The listing builds one solid part. Answer for the finished solid, in the listing's coordinates (mm). Face numbers are marked on the shaded views. A direction names the side the tool comes from. Coordinates: 2 decimals unless noted, no trailing zeros. Loops run counter-clockwise (first coordinate to the right, second up) from the corner with the lowest first, then second, coordinate; pieces in that order, holes last. Notation, with made-up numbers: M -31.5,-22 L -22.5,-22 A34 cw -22.5,12 Z; hole C -34,-24 d1. An arc over 180 degrees is marked long. Answer as a JSON object with one key per item and string values. Group by question number.
1. Determine the mould class of the marked faces 3, 4 and 5 for opening direction Y: released by +Y, released by -Y, zero draft, split by the parting line, or undercut.
2. For the marked faces 1 and 2, determine the directions among +Z, -Z, +X, -X, +Y, -Y from which every point of the face is accessible in a straight line to the end or side of a thin tool.
3. A cutting plane is placed at A-A on z = 10. Give the vertices of the cut face in (x, y), and give its area (4 significant figures).
4. A cutting plane is placed at C-C on y = 10. Give the vertices of the cut face in (x, z), and give its area (3 significant figures).
5. Straight lines are drawn through the part: L1, parallel to X at y = 6, z = 3.75; L2, parallel to Y at x = 67.5, z = 9.5; L3, parallel to Z at x = 10, y = 3.5. For each, find the intervals that lie inside material, in ascending order.
6. A cutting plane is placed at B-B on x = 45. Give the vertices of the cut face in (y, z), and give its area (3 significant figures).
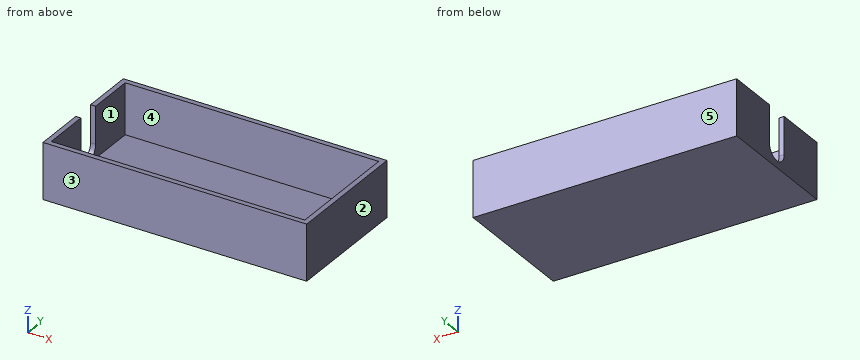
from build123d import *

# Parameters (mm, degrees)
ESQUISSE1_W             = 75
ESQUISSE1_H             = 35
BOSS_EXTRU_1_DEPTH      = 15
COQUE1_T                = 1.5
ENL_V_MAT_EXTRU_1_DEPTH = 15


with BuildPart() as part:
    # Esquisse1 → Boss.-Extru.1 (new body)
    with BuildSketch(Plane.XY):
        with Locations((37.5, 17.5)):
            Rectangle(ESQUISSE1_W, ESQUISSE1_H)
    extrude(amount=BOSS_EXTRU_1_DEPTH)

    # Coque1
    coque1_openings = [part.faces().sort_by_distance(p)[0] for p in [
        (37.5, 17.5, 15),
    ]]
    offset(amount=COQUE1_T, openings=coque1_openings, kind=Kind.INTERSECTION)

    # Esquisse2 → Enlèv. mat.-Extru.1 (cut)
    with BuildSketch(Plane.ZY.offset(1.5)):
        with BuildLine():
            Line((4, 21), (15.502923277, 21))
            ThreePointArc((15.502923277, 21), (19.002923277, 17.5), (15.502923277, 14))
            Line((15.502923277, 14), (4, 14))
            ThreePointArc((4, 14), (0.5, 17.5), (4, 21))
        make_face()
    extrude(amount=-ENL_V_MAT_EXTRU_1_DEPTH, mode=Mode.SUBTRACT)


solid = part.part
From the geometry:
{
 "1": {"face 3": "released by -Y", "face 4": "undercut", "face 5": "released by +Y"},
 "2": {"face 1": "+Z", "face 2": "+Z, -Z, +X, +Y, -Y"},
 "3": {"outline": "M -1.5,-1.5 L 76.5,-1.5 L 76.5,36.5 L -1.5,36.5 L -1.5,21 L 0,21 L 0,35 L 75,35 L 75,0 L 0,0 L 0,14 L -1.5,14 Z", "area": "328.5 mm²"},
 "4": {"outline": "M -1.5,-1.5 L 76.5,-1.5 L 76.5,15 L 75,15 L 75,0 L 0,0 L 0,15 L -1.5,15 Z", "area": "162 mm²"},
 "5": {"L1": "x = -1.5 to 0, 75 to 76.5", "L2": "y = -1.5 to 0, 35 to 36.5", "L3": "z = -1.5 to 0"},
 "6": {"outline": "M -1.5,-1.5 L 36.5,-1.5 L 36.5,15 L 35,15 L 35,0 L 0,0 L 0,15 L -1.5,15 Z", "area": "102 mm²"}
}
